```python
from build123d import *

# Parameters (mm, degrees)
SKIZZE1_W                       = 120
SKIZZE1_H                       = 8
SKIZZE1_R                       = 1.75
AUFSATZ_LINEAR_AUSTRAGEN1_DEPTH = 8
SKIZZE2_R                       = 1.75
SCHNITT_LINEAR_AUSTRAGEN1_DEPTH = 62.05735009


with BuildPart() as part:
    # Skizze1 → Aufsatz-Linear austragen1 (new body)
    with BuildSketch(Plane.XY):
        Rectangle(SKIZZE1_W, SKIZZE1_H)
        with Locations((-35, 0)):
            Circle(SKIZZE1_R, mode=Mode.SUBTRACT)
        with Locations((35, 0)):
            Circle(SKIZZE1_R, mode=Mode.SUBTRACT)
    extrude(amount=AUFSATZ_LINEAR_AUSTRAGEN1_DEPTH)

    # Skizze2 → Schnitt-Linear austragen1 (cut, through all)
    with BuildSketch(Plane(origin=(0, 4, 0), x_dir=(1, 0, 0), z_dir=(0, 1, 0))):
        with Locations(Location((53, -4, 0), (0, 0, 270))):
            Circle(SKIZZE2_R)
        with Locations(Location((-53, -4, 0), (0, 0, 90))):
            Circle(SKIZZE2_R)
        with Locations(Location((0, -4, 0), (0, 0, 270))):
            Circle(SKIZZE2_R)
    extrude(amount=-SCHNITT_LINEAR_AUSTRAGEN1_DEPTH, mode=Mode.SUBTRACT)


solid = part.part
```
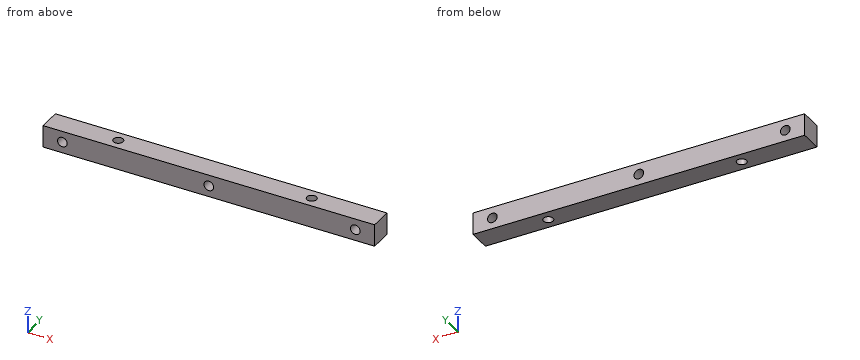
Source: CAD feature listing. Evaluate the final solid. Frame: model axes, mm. Round coordinates to 2 decimals unless told otherwise and drop trailing zeros. Write each loop counter-clockwise with the first axis right and the second up, starting at its lowest first coordinate (ties: lowest second). Pieces come first, ordered by that corner, then holes. Notation, with made-up numbers: M 84.25,41.25 L 142.25,41.25 A13 ccw 142.25,45.25 Z; hole C 16,-7.5 d2. An arc over 180 degrees is marked long. Use CSV: the item, a comma, the result in double quotes. Start each with the question number.
Q1. Cut plane B-B on z = 4. Output: boundary loops of the cut face in (x, y).
Q2. Cut plane A-A on y = 0. Output: boundary loops of the cut face in (x, z).
Q3. Cut plane C-C on x = -53. Output: boundary loops of the cut face in (y, z), plus the area to 3 significant figures.
Q4. Line query: line 1 (X direction, y = 2.25, z = 4); line 2 (X direction, y = 0.25, z = 4); line 3 (Y direction, x = 35, z = 6.25). Output: solid intervals per line, ascending. Write a range as from..to.
Results found:
1,outline,"M -60,-4 L -54.75,-4 L -54.75,4 L -60,4 Z; M -51.25,-4 L -1.75,-4 L -1.75,4 L -51.25,4 Z; M 1.75,-4 L 51.25,-4 L 51.25,4 L 1.75,4 Z; M 54.75,-4 L 60,-4 L 60,4 L 54.75,4 Z; hole C -35,0 d3.5; hole C 35,0 d3.5"
2,outline,"M -60,0 L -36.75,0 L -36.75,8 L -60,8 Z; M -33.25,0 L 33.25,0 L 33.25,8 L -33.25,8 Z; M 36.75,0 L 60,0 L 60,8 L 36.75,8 Z; hole C -53,4 d3.5; hole C 0,4 d3.5; hole C 53,4 d3.5"
3,outline,"M -4,0 L 4,0 L 4,2.25 L -4,2.25 Z; M -4,5.75 L 4,5.75 L 4,8 L -4,8 Z"
3,area,"36.0 mm^2"
4,line 1,"-60..-54.75, -51.25..-1.75, 1.75..51.25, 54.75..60"
4,line 2,"-60..-54.75, -51.25..-36.73, -33.27..-1.75, 1.75..33.27, 36.73..51.25, 54.75..60"
4,line 3,"-4..-1.75, 1.75..4"
